Could you check a few things on this model? Use its own coordinates, in mm. A direction names the side the tool comes from. Give positions to 0.01 mm unless a question says otherwise; leave off trailing zeros. Write each loop counter-clockwise with the first axis right and the second up, starting at its lowest first coordinate (ties: lowest second). Pieces come first, ordered by that corner, then holes. Notation, with made-up numbers: (-12, 7.25) - (15, 7.25) arc R19 cw to (15, 36.25) - close; hole circle Ø5 at (-0.75, 37). An arc over 180 degrees is marked (long way). Answer in a Markdown table with one row per item.
from build123d import *

# Parameters (mm, degrees)
F1_DEPTH = 36.5


with BuildPart() as f1:
    # F0 (on Top) → F1 (new body)
    with BuildSketch(Plane.XY):
        Polygon((16.5, 0), (0, 0), (0, 48), (16.5, 48), (16.5, 43), (17.7, 43), (17.7, 49.2), (-1.2, 49.2), (-1.2, -1.2), (17.7, -1.2), (17.7, 2.5), (16.5, 2.5), align=None)
    extrude(amount=-F1_DEPTH)


solid = f1.part
1) Imagine slicing it at D-D (y = 25.5). List the corners of the cut face in (x, z) for me, then the cut area to 3 significant figures.
Check values:
| item | result |
|---|---|
| outline | (-1.2, -36.5) - (0, -36.5) - (0, 0) - (-1.2, 0) - close |
| area | 43.8 mm2 |
2) Imagine slicing it at A-A (x = 2.75). List the corners of the cut face in (y, z) for me.
Check values:
| item | result |
|---|---|
| outline | (-1.2, -36.5) - (0, -36.5) - (0, 0) - (-1.2, 0) - close; (48, -36.5) - (49.2, -36.5) - (49.2, 0) - (48, 0) - close |
3) Imagine slicing it at B-B (y = 46.5). List the corners of the cut face in (x, z) for me.
Check values:
| item | result |
|---|---|
| outline | (-1.2, -36.5) - (0, -36.5) - (0, 0) - (-1.2, 0) - close; (16.5, -36.5) - (17.7, -36.5) - (17.7, 0) - (16.5, 0) - close |
4) Will this pin go through, and if not, where does the flat tip stop? P1, Ø2, axis at y = 38.5, z = -11.5, coming from the +X side.
Check values:
| item | result |
|---|---|
| P1 | stops at x = 0 |
5) On a 3-axis mill with a long thin cutter (end or side, diameter ignored), from which of +Z, -Z, +X, -X, +Y, -Y can I reach the whole of each face in a straight line? I mean faces 1 (the face through (16.5, 46, -18)), 2 (the face through (17, 2.5, -18)), 3 (the face through (-0.2, 24.1, 0)). Say none if no direction works.
Check values:
| item | result |
|---|---|
| face 1 | +Z, -Z |
| face 2 | +Z, -Z, +X |
| face 3 | +Z, +X, -X, +Y, -Y |
6) Imagine slicing it at C-C (z = -10). List the corners of the cut face in (x, y) for me, then the cut area to 3 significant figures.
Check values:
| item | result |
|---|---|
| outline | (-1.2, -1.2) - (17.7, -1.2) - (17.7, 2.5) - (16.5, 2.5) - (16.5, 0) - (0, 0) - (0, 48) - (16.5, 48) - (16.5, 43) - (17.7, 43) - (17.7, 49.2) - (-1.2, 49.2) - close |
| area | 112 mm2 |
7) We'd pull the mould along Y, two halves only. Please class faces 4 (the face through (17, 43, -18)), 5 (the face through (17.7, 1, -18)), 6 (the face through (8, 49.2, -18)), 7 (the face through (8, -1.2, -18)): +Y half, -Y half, draft (parallel to the pull), parting line (faces both ways), or undercut.
Check values:
| item | result |
|---|---|
| face 4 | undercut |
| face 5 | draft |
| face 6 | +Y half |
| face 7 | -Y half |
8) If I drill on line 1 (Y direction, x = 8.75, z = -4.5); line 2 (X direction, y = 44.5, z = -20); line 3 (X direction, y = 37, z = -23.5), over which ranges is the centre line in solid material (lowest first)?
Check values:
| item | result |
|---|---|
| line 1 | y = -1.2 to 0, 48 to 49.2 |
| line 2 | x = -1.2 to 0, 16.5 to 17.7 |
| line 3 | x = -1.2 to 0 |
